from build123d import *

# Parameters (mm, degrees)
F0_R     = 11
F1_DEPTH = 2
F2_R     = 3.5
F3_DEPTH = 6
F4_R     = 2
F5_DEPTH = 6
F6_R     = 1.99999


# Not quite as in the source:
# - a fillet or chamfer is up to 0.001 mm smaller than in the source, because OpenCascade refuses the exact size


with BuildPart() as f1:
    # F0 (on Top) → F1 (new body)
    with BuildSketch(Plane.XY):
        Circle(F0_R)
    extrude(amount=F1_DEPTH)

    # F2 (on face) → F3 (join)
    with BuildSketch(Plane.XY.offset(2)):
        Circle(F2_R)
    extrude(amount=F3_DEPTH)

    # F4 (on face) → F5 (cut)
    with BuildSketch(Plane.XY.offset(8)):
        Circle(F4_R)
    extrude(amount=-F5_DEPTH, mode=Mode.SUBTRACT)

    # F6 (radius 2 in the source; OpenCascade refuses exactly that, so slightly less here)
    f6_edges = [f1.edges().sort_by_distance(p)[0] for p in [
        (-11, 0, 0),
    ]]
    fillet(f6_edges, radius=F6_R)


solid = f1.part
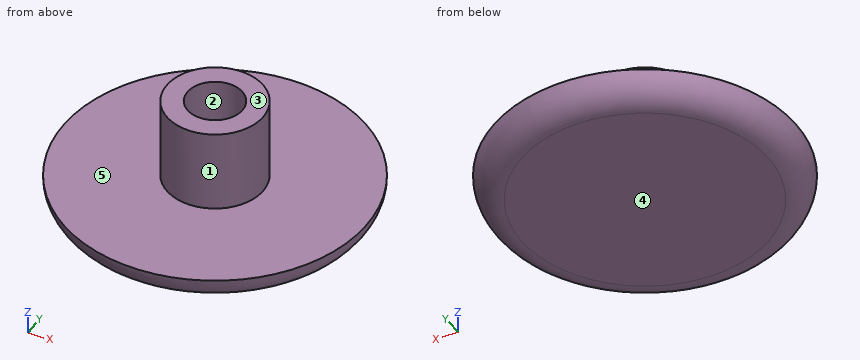
Here's how the part is built. I have some questions about the finished solid (model axes, mm). Face numbers are marked on the shaded views. A direction names the side the tool comes from. Give positions to 0.01 mm unless a question says otherwise; leave off trailing zeros. Order: outer loops, then holes, each group sorted by start corner. A loop starts at its lowest first (then second) coordinate and runs counter-clockwise, first axis right, second up. Notation, with made-up numbers: M -9,-24 L 20,-24 A19 cw 20,-20 Z; hole C 69,70 d6. An arc over 180 degrees is marked long. Answer as a JSON object with one key per item and string values. Group by question number.
1) We'd pull the mould along Y, two halves only. Please class the marked faces 1, 2 and 3: pulls with the +Y half, pulls with the -Y half, needs draft (parallel to the pull), parting line crosses it, or undercut.
2) Please list where these lines run through material, in increasing order: L1, parallel to Y at x = 0, z = 5.7; L2, parallel to Z at x = 7.5, y = 1; L3, parallel to Y at x = 0.5, z = 4. Write a range as [from, to].
3) I'm going to push flat-ended pins straight in: pin 1 Ø8 at (x, y) = (9, -7) entering from +Z; pin 2 Ø2 at (y, z) = (-0.5, 4) entering from +X. Where does each tip first touch, or does it pass through?
4) Suppose I cut it at B-B, the plane z = 7. Write out the boundary of the cut face in (x, y).
5) On a 3-axis mill with a long thin cutter (end or side, diameter ignored), from which of +Z, -Z, +X, -X, +Y, -Y can I reach the whole of each face in a straight line? I mean the marked faces 4 and 5. Say none if no direction works.
Results found:
{
 "1": {"face 1": "parting line crosses it", "face 2": "undercut", "face 3": "needs draft"},
 "2": {"L1": "[-3.5, -2], [2, 3.5]", "L2": "[0, 2]", "L3": "[-3.46, -1.94], [1.94, 3.46]"},
 "3": {"pin 1": "z = 2", "pin 2": "x = 3.5"},
 "4": {"outline": "C 0,0 d7; hole C 0,0 d4"},
 "5": {"face 4": "-Z, +X, -X, +Y, -Y", "face 5": "+Z"}
}
